Input: part model. Units: mm. Frame: model coordinates. Face numbers are marked on the shaded views. A direction names the side the tool comes from. Coordinates: 2 decimals unless noted, no trailing zeros. Write each loop counter-clockwise with the first axis right and the second up, starting at its lowest first coordinate (ties: lowest second). Pieces come first, ordered by that corner, then holes. Notation, with made-up numbers: (71, -37) -> (94, -37) arc R24 ccw to (94, -27) -> close; hole circle Ø9 at (-31.75, 40). An arc over 180 degrees is marked (long way). One line per question, with ' | ' between items. Start each with the question number.
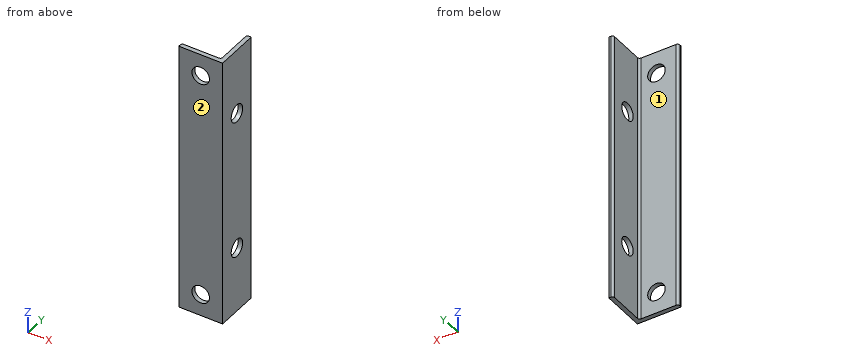
```python
from build123d import *

# Parameters (mm, degrees)
BOSS_EXTRUDE1_DEPTH = 49.2125
SKETCH3_R           = 3.175
CUT_EXTRUDE1_DEPTH  = 16.875
CUT_EXTRUDE2_REACH  = 17.875
SKETCH4_R           = 3.175


with BuildPart() as part:
    # Sketch2 → Boss-Extrude1 (new body, symmetric)
    with BuildSketch(Plane.XY):
        with BuildLine():
            Line((-7.9375, 0), (7.9375, 0))
            Line((7.9375, 0), (7.9375, 15.875))
            Line((7.9375, 15.875), (7.14375, 15.875))
            ThreePointArc((7.14375, 15.875), (6.582483992, 15.642516008), (6.35, 15.08125))
            Line((6.35, 15.08125), (6.35, 2.38125))
            ThreePointArc((6.35, 2.38125), (6.117516008, 1.819983992), (5.55625, 1.5875))
            Line((5.55625, 1.5875), (-7.14375, 1.5875))
            ThreePointArc((-7.14375, 1.5875), (-7.705016008, 1.355016008), (-7.9375, 0.79375))
            Line((-7.9375, 0.79375), (-7.9375, 0))
        make_face()
    extrude(amount=BOSS_EXTRUDE1_DEPTH, both=True)

    # Sketch3 → Cut-Extrude1 (cut, through all)
    with BuildSketch(Plane(origin=(7.9375, 0, 0), x_dir=(0, 0, -1), z_dir=(1, 0, 0))):
        with Locations((-25.4, 7.9375)):
            Circle(SKETCH3_R)
        with Locations((25.4, 7.9375)):
            Circle(SKETCH3_R)
    extrude(amount=-CUT_EXTRUDE1_DEPTH, mode=Mode.SUBTRACT)

    # Sketch4 → Cut-Extrude2 (cut, up to next)
    with BuildSketch(Plane.XZ, mode=Mode.PRIVATE) as cut_extrude2_sk1:
        with Locations((0, -41.275)):
            Circle(SKETCH4_R)
    cut_extrude2_tool1 = extrude(cut_extrude2_sk1.sketch, amount=-CUT_EXTRUDE2_REACH, mode=Mode.PRIVATE) & part.part
    add(cut_extrude2_tool1.solids().sort_by_distance((0, 0, -41.275))[0], mode=Mode.SUBTRACT)
    # Sketch4 → Cut-Extrude2 (cut, up to next)
    with BuildSketch(Plane.XZ, mode=Mode.PRIVATE) as cut_extrude2_sk2:
        with Locations((0, 41.275)):
            Circle(SKETCH4_R)
    cut_extrude2_tool2 = extrude(cut_extrude2_sk2.sketch, amount=-CUT_EXTRUDE2_REACH, mode=Mode.PRIVATE) & part.part
    add(cut_extrude2_tool2.solids().sort_by_distance((0, 0, 41.275))[0], mode=Mode.SUBTRACT)


solid = part.part
```
1) Access query for the marked faces 1 and 2. Directions: +Z, -Z, +X, -X, +Y, -Y. A direction counts if a zero-diameter tool reaches every point of the face in a straight line with its end or side. Return the directions, or none.
2) First-contact query: P1, Ø4, axis at x = -1.5, z = -22, coming from the +Y side; P2, Ø4, axis at y = 8.5, z = 15.5, coming from the -X side. Flat tips, straight axial feed; report the tip coordinate or a pass-through.
3) Section D-D, the plane y = 14.25. Return loops of the section in (x, z), then the cut area to 3 significant figures.
4) Section B-B, the plane x = 0. Return loops of the section in (y, z), then the cut area to 3 significant figures.
5) Ray query, line 1 (Z direction, x = 6.5, y = 8.25); line 2 (Z direction, x = -0.75, y = 0.5); line 3 (Y direction, x = 7.45, z = 25.4) (1 decimal). Return the intervals inside material, ascending.
Answer block:
1) face 1: +Z, -Z, -X, +Y | face 2: +Z, -Z, +X, -X, -Y
2) P1: stops at y = 1.59 | P2: stops at x = 6.35
3) outline: (6.35, -49.21) -> (7.94, -49.21) -> (7.94, 49.21) -> (6.35, 49.21) -> close | area: 156 mm2
4) outline: (0, -49.21) -> (1.59, -49.21) -> (1.59, -44.45) -> (0, -44.45) -> close; (0, -38.1) -> (1.59, -38.1) -> (1.59, 38.1) -> (0, 38.1) -> close; (0, 44.45) -> (1.59, 44.45) -> (1.59, 49.21) -> (0, 49.21) -> close | area: 136 mm2
5) line 1: z = -49.21 to -28.56, -22.24 to 22.24, 28.56 to 49.21 | line 2: z = -49.21 to -44.36, -38.19 to 38.19, 44.36 to 49.21 | line 3: y = 0 to 4.8, 11.1 to 15.9
